Geometry: final body of the model. Coordinates: model frame, mm. A direction names the side the tool comes from. Give positions to 0.01 mm unless a question says otherwise; leave off trailing zeros. Order: outer loops, then holes, each group sorted by start corner. A loop starts at its lowest first (then second) coordinate and runs counter-clockwise, first axis right, second up. Notation, with made-up numbers: (23.25, 63) - (70.25, 63) arc R6 cw to (70.25, 74) - close; hole circle Ø10 at (-23.5, -14). An arc over 180 degrees is marked (long way). Use one line per item in the form item = value.
from build123d import *

# Parameters (mm, degrees)
SKETCH1_R               = 1.5
SKETCH1_W               = 28
SKETCH1_H               = 54
BOSS_EXTRUDE1_DEPTH     = 8
SKETCH4_W               = 46
SKETCH4_H               = 6
CUT_EXTRUDE1_DEPTH      = 1
CUT_EXTRUDE1_DEPTH_BACK = 29
SKETCH5_R               = 4
CUT_EXTRUDE2_DEPTH      = 1
CUT_EXTRUDE2_DEPTH_BACK = 29


with BuildPart() as part:
    # Sketch1 → Boss-Extrude1 (new body)
    with BuildSketch(Plane(origin=(0, 12.242650433, 0), x_dir=(1, 0, 0), z_dir=(0, 1, 0))):
        Polygon((-49.268515773, 16.802150236), (-49.268515773, 15.802150236), (-21.268515773, 15.802150236), (-21.268515773, 16.802150236), (-21.268515773, 17.094050992), (-21.268515773, 24.510249479), (-21.268515773, 24.802150236), (-21.268515773, 30.802150236), (-49.268515773, 30.802150236), (-49.268515773, 24.802150236), (-49.268515773, 24.510249479), (-49.268515773, 17.094050992), align=None)
        with Locations((-45.268515773, 27.302150236)):
            Circle(SKETCH1_R, mode=Mode.SUBTRACT)
        with Locations((-25.268515773, 27.302150236)):
            Circle(SKETCH1_R, mode=Mode.SUBTRACT)
        with Locations((-35.268515773, -11.197849764)):
            Rectangle(SKETCH1_W, SKETCH1_H)
        Polygon((-49.268515773, -47.197849764), (-49.268515773, -53.197849764), (-21.268515773, -53.197849764), (-21.268515773, -47.197849764), (-21.268515773, -46.905949008), (-21.268515773, -39.489750521), (-21.268515773, -39.197849764), (-21.268515773, -38.197849764), (-49.268515773, -38.197849764), (-49.268515773, -39.197849764), (-49.268515773, -39.489750521), (-49.268515773, -46.905949008), align=None)
        with Locations((-45.268515773, -49.697849764)):
            Circle(SKETCH1_R, mode=Mode.SUBTRACT)
        with Locations((-25.268515773, -49.697849764)):
            Circle(SKETCH1_R, mode=Mode.SUBTRACT)
    extrude(amount=-BOSS_EXTRUDE1_DEPTH)

    # Sketch4 → Cut-Extrude1 (cut, two sides)
    with BuildSketch(Plane(origin=(-21.268515773, 0, 0), x_dir=(0, 0, -1), z_dir=(1, 0, 0))) as cut_extrude1_sk:
        with Locations((-15.197849764, 9.242650433)):
            Rectangle(SKETCH4_W, SKETCH4_H)
    extrude(amount=CUT_EXTRUDE1_DEPTH, mode=Mode.SUBTRACT)
    extrude(cut_extrude1_sk.sketch, amount=-CUT_EXTRUDE1_DEPTH_BACK, mode=Mode.SUBTRACT)

    # Sketch5 → Cut-Extrude2 (cut, two sides)
    with BuildSketch(Plane(origin=(-21.268515773, 0, 0), x_dir=(0, 0, -1), z_dir=(1, 0, 0))) as cut_extrude2_sk:
        with Locations((-43.197849764, 13.742650433)):
            Circle(SKETCH5_R)
        with Locations((20.802150236, 13.742650433)):
            Circle(SKETCH5_R)
    extrude(amount=CUT_EXTRUDE2_DEPTH, mode=Mode.SUBTRACT)
    extrude(cut_extrude2_sk.sketch, amount=-CUT_EXTRUDE2_DEPTH_BACK, mode=Mode.SUBTRACT)


solid = part.part
(1) Ray query, line 1 along Z through (x, y) = (-29, 8.75); line 2 along X through (y, z) = (8, 49); line 3 along Y through (x, z) = (-45.5, 43). Return the intervals inside material, ascending.
Computed values:
line_1 = -30.8 to -7.8, 38.2 to 53.2
line_2 = -49.27 to -46.6, -43.94 to -26.6, -23.94 to -21.27
line_3 = 4.24 to 9.75
(2) Cut plane D-D on z = 27.5. Output: boundary loops of the cut face in (x, y).
Computed values:
outline = (-49.27, 4.24) - (-21.27, 4.24) - (-21.27, 6.24) - (-49.27, 6.24) - close
(3) Cut plane B-B on x = -46. Output: boundary loops of the cut face in (y, z), plus the area to 3 significant figures.
Computed values:
outline = (4.24, -30.8) - (12.24, -30.8) - (12.24, -28.61) - (4.24, -28.61) - close; (4.24, -25.99) - (12.24, -25.99) - (12.24, -24.51) arc R4 cw to (12.24, -17.09) - (12.24, -7.8) - (6.24, -7.8) - (6.24, 38.2) - (12.24, 38.2) - (12.24, 39.49) arc R4 cw to (12.24, 46.91) - (12.24, 48.39) - (4.24, 48.39) - close; (4.24, 51.01) - (12.24, 51.01) - (12.24, 53.2) - (4.24, 53.2) - close
area = 327 mm²
(4) Cut plane A-A on y = 10.5. Output: boundary loops of the cut face in (x, z).
Computed values:
outline = (-49.27, -30.8) - (-21.27, -30.8) - (-21.27, -23.14) - (-49.27, -23.14) - close; (-49.27, -18.46) - (-21.27, -18.46) - (-21.27, -7.8) - (-49.27, -7.8) - close; (-49.27, 38.2) - (-21.27, 38.2) - (-21.27, 40.86) - (-49.27, 40.86) - close; (-49.27, 45.54) - (-21.27, 45.54) - (-21.27, 53.2) - (-49.27, 53.2) - close; hole circle Ø3 at (-45.27, -27.3); hole circle Ø3 at (-45.27, 49.7); hole circle Ø3 at (-25.27, -27.3); hole circle Ø3 at (-25.27, 49.7)
(5) Pull-direction query (X, two-part tool) for faces 3 (the face through (-21.269, 6, 12)), 4 (the face through (-43.838, 8.299, 49.247)), 5 (the face through (-35, 8, 53.198)); classes: released by +X, released by -X, zero draft, split by the parting line, or undercut.
Computed values:
face_3 = released by +X
face_4 = undercut
face_5 = zero draft
(6) Cut plane C-C on x = -42. Output: boundary loops of the cut face in (y, z).
Computed values:
outline = (4.24, -30.8) - (12.24, -30.8) - (12.24, -24.51) arc R4 cw to (12.24, -17.09) - (12.24, -7.8) - (6.24, -7.8) - (6.24, 38.2) - (12.24, 38.2) - (12.24, 39.49) arc R4 cw to (12.24, 46.91) - (12.24, 53.2) - (4.24, 53.2) - close
(7) Contact query for a flat-ended pin moving along its axis: pin 1 Ø10 at (x, z) = (-38.5, 3) entering from +Y. Output: stop coordinate, or through.
Computed values:
pin_1 = 6.24
(8) Reachability of faces 1 (the face through (-35, 9, -7.802)), 2 (the face through (-49.269, 6, 11)) from +Z, -Z, +X, -X, +Y, -Y: full face, straight path, thin tool, end or side. Return the list, or none.
Computed values:
face_1 = +X, -X, +Y
face_2 = +Z, -Z, -X, +Y, -Y
